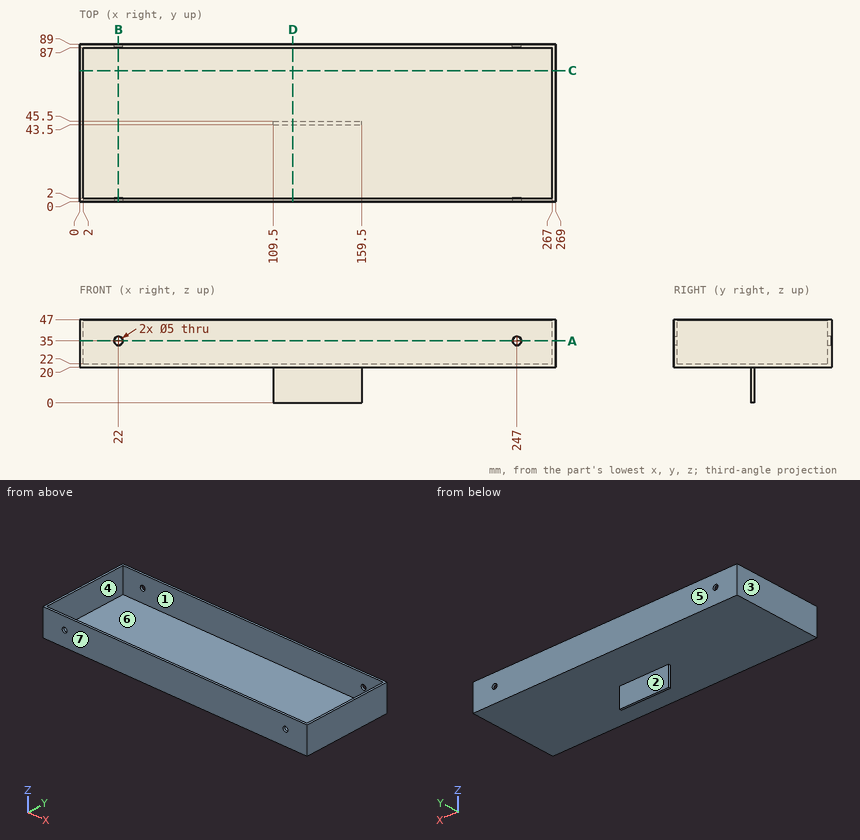
Source: three-view drawing plus pictorial views. Frame: mm from the lowest corner of the part. A direction names the side the tool comes from. Round coordinates to 2 decimals unless told otherwise and drop trailing zeros. Loops run counter-clockwise (first coordinate to the right, second up) from the corner with the lowest first, then second, coordinate; pieces in that order, holes last.
Q1. Access query for the marked faces 1, 2 and 3. Directions: +Z, -Z, +X, -X, +Y, -Y. A direction counts if a zero-diameter tool reaches every point of the face in a straight line with its end or side. Return the directions, or none.
Q2. Section A-A on z = 35. Return loops of the section in (x, y).
Q3. Pin query (flat end, axial travel): P1, Ø3, axis at x = 247, z = 35, coming from the +Y side; P2, Ø10, axis at x = 139, z = 6, coming from the +Y side; P3, Ø2, axis at y = 45, z = 10.5, coming from the -X side; P4, Ø8, axis at x = 188.5, y = 11, coming from the -Z side. Return the tip coordinate at first contact, or that it passes through.
Q4. Pull-direction query (Y, two-part tool) for the marked faces 4, 5, 6 and 7; classes: released by +Y, released by -Y, zero draft, split by the parting line, or undercut.
Q5. Section D-D on x = 120.5. Return loops of the section in (y, z).
Q6. Material intervals for L1, parallel to X at y = 0.95, z = 35; L2, parallel to Y at x = 54, z = 45.5; L3, parallel to X at y = 43.5, z = 22.5, sorted ascending.
Q7. Section C-C on y = 74. Return loops of the section in (x, z).
Q8. Section B-B on x = 22. Return loops of the section in (y, z).
Evaluation:
1. face 1: +Z
1. face 2: -Z, +X, -X, +Y
1. face 3: +Z, -Z, -X, +Y, -Y
2. outline: (0, 0) - (19.5, 0) - (19.5, 2) - (2, 2) - (2, 87) - (19.5, 87) - (19.5, 89) - (0, 89) - close; (24.5, 0) - (244.5, 0) - (244.5, 2) - (24.5, 2) - close; (24.5, 87) - (244.5, 87) - (244.5, 89) - (24.5, 89) - close; (249.5, 0) - (269, 0) - (269, 89) - (249.5, 89) - (249.5, 87) - (267, 87) - (267, 2) - (249.5, 2) - close
3. P1: passes through
3. P2: stops at y = 45.5
3. P3: stops at x = 109.5
3. P4: stops at z = 20
4. face 4: undercut
4. face 5: released by +Y
4. face 6: undercut
4. face 7: released by -Y
5. outline: (0, 20) - (43.5, 20) - (43.5, 0) - (45.5, 0) - (45.5, 20) - (89, 20) - (89, 47) - (87, 47) - (87, 22) - (2, 22) - (2, 47) - (0, 47) - close
6. L1: x = 0 to 19.5, 24.5 to 244.5, 249.5 to 269
6. L2: y = 0 to 2, 87 to 89
6. L3: x = 0 to 2, 267 to 269
7. outline: (0, 20) - (269, 20) - (269, 47) - (267, 47) - (267, 22) - (2, 22) - (2, 47) - (0, 47) - close
8. outline: (0, 20) - (89, 20) - (89, 32.5) - (87, 32.5) - (87, 22) - (2, 22) - (2, 32.5) - (0, 32.5) - close; (0, 37.5) - (2, 37.5) - (2, 47) - (0, 47) - close; (87, 37.5) - (89, 37.5) - (89, 47) - (87, 47) - close
